```python
from build123d import *

# Parameters (mm, degrees)
F0_W     = 125.222
F0_H     = 98.425
F0_W_2   = 99.822
F0_H_2   = 85.979
F0_R     = 1.27
F0_R_2   = 36.5125
F1_DEPTH = 19.05
F2_W     = 559.8626548463
F2_H     = 85.725
F3_DEPTH = 12.7
F2_W_2   = 125.222
F2_R     = 1.27
F2_R_2   = 36.5125
F4_DEPTH = 12.7


with BuildPart() as f1:
    # F0 (on Front) → F1 (new body)
    with BuildSketch(Plane.XZ):
        with Locations((-326.1520862579, 56.1317810915)):
            Rectangle(F0_W, F0_H)
        with Locations((-326.1520862579, 56.1317810915)):
            Rectangle(F0_W_2, F0_H_2, mode=Mode.SUBTRACT)
        with Locations((-326.1520862579, 56.1317810915)):
            Rectangle(F0_W_2, F0_H_2)
        with Locations((-372.7610862579, 16.7490810915)):
            Circle(F0_R, mode=Mode.SUBTRACT)
        with Locations((-279.5430862579, 16.7617810915)):
            Circle(F0_R, mode=Mode.SUBTRACT)
        with Locations((-326.1520862579, 56.1317810915)):
            Circle(F0_R_2, mode=Mode.SUBTRACT)
        with Locations((-372.7610862579, 95.4890810915)):
            Circle(F0_R, mode=Mode.SUBTRACT)
        with Locations((-279.5430871231, 95.5017810915)):
            Circle(F0_R, mode=Mode.SUBTRACT)
    extrude(amount=F1_DEPTH)

    # F2 (on face) → F3 (cut)
    with BuildSketch(Plane.XZ.offset(19.05)):
        with Locations((-149.6497262269, 56.1317810915)):
            Rectangle(F2_W, F2_H)
    extrude(amount=-F3_DEPTH, mode=Mode.SUBTRACT)

    # F2 (on face) → F4 (cut)
    with BuildSketch(Plane.XZ.offset(19.05)):
        with Locations((-326.1520862579, 56.1317810915)):
            Rectangle(F2_W_2, F2_H)
        with Locations((-372.7610862579, 16.7490810915)):
            Circle(F2_R, mode=Mode.SUBTRACT)
        with Locations((-279.5430862579, 16.7617810915)):
            Circle(F2_R, mode=Mode.SUBTRACT)
        with Locations((-326.1520862579, 56.1317810915)):
            Circle(F2_R_2, mode=Mode.SUBTRACT)
        with Locations((-372.7610862579, 95.4890810915)):
            Circle(F2_R, mode=Mode.SUBTRACT)
        with Locations((-279.5430871231, 95.5017810915)):
            Circle(F2_R, mode=Mode.SUBTRACT)
    extrude(amount=-F4_DEPTH, mode=Mode.SUBTRACT)


solid = f1.part
```
Geometry check sheet. Reference: the model listing, model coordinates, mm. A direction names the side the tool comes from. Give positions to 0.01 mm unless a question says otherwise; leave off trailing zeros. Write each loop counter-clockwise with the first axis right and the second up, starting at its lowest first coordinate (ties: lowest second). Pieces come first, ordered by that corner, then holes. Notation, with made-up numbers: (-29.75, 12.25) - (-25.75, 12.25) arc R27 ccw to (-25.75, 31.25) - close; hole circle Ø9 at (30, 0). An arc over 180 degrees is marked (long way). Use a Markdown table: item, result.
Q1. Section check B-B, the plane z = 78. Enter the section's corners in (x, y), then the cut area to 3 significant figures.
Computed:
| item | result |
|---|---|
| outline | (-388.76, -6.35) - (-355.39, -6.35) - (-355.39, 0) - (-388.76, 0) - close; (-296.91, -6.35) - (-263.54, -6.35) - (-263.54, 0) - (-296.91, 0) - close |
| area | 424 mm² |
Q2. Section check C-C, the plane x = -303.5. Enter the section's corners in (y, z), then the cut area to 3 significant figures.
Computed:
| item | result |
|---|---|
| outline | (-19.05, 6.92) - (0, 6.92) - (0, 27.5) - (-6.35, 27.5) - (-6.35, 13.27) - (-19.05, 13.27) - close; (-19.05, 98.99) - (-6.35, 98.99) - (-6.35, 84.77) - (0, 84.77) - (0, 105.34) - (-19.05, 105.34) - close |
| area | 423 mm² |
Q3. Draft check along X on faces 3 (the face through (-292.424, -3.131, 42.147)), 4 (the face through (-388.763, -5, 55)), 5 (the face through (-327, -19.05, 102)). Enter one of: pulls with the +X half, pulls with the -X half, needs draft (parallel to the pull), parting line crosses it, or undercut.
Computed:
| item | result |
|---|---|
| face 3 | undercut |
| face 4 | pulls with the -X half |
| face 5 | needs draft |
Q4. Thickness scan on L1, parallel to Z at x = -322, y = -9.5; L2, parallel to X at y = -5.5, z = 16; L3, parallel to Y at x = -271.5, z = 95. Record the ranges inside material, lowest first. Write a range as [from, to].
Computed:
| item | result |
|---|---|
| L1 | z = [6.92, 13.27], [98.99, 105.34] |
| L2 | x = [-388.76, -373.79], [-371.74, -280.56], [-278.53, -263.54] |
| L3 | y = [-6.35, 0] |
Q5. Go/stop test with flat-tipped pins: P1, Ø3, axis at y = -9, z = 72.5, coming from the -X side; P2, Ø8, axis at x = -371, z = 21, coming from the -Y side. Record where each tip stops, or that it passes through.
Computed:
| item | result |
|---|---|
| P1 | passes through |
| P2 | stops at y = -6.35 |
Q6. Set-up check for faces 1 (the face through (-327, -13, 13.269)), 2 (the face through (-327, -19.05, 10)): record each of +Z, -Z, +X, -X, +Y, -Y from which the full face is reachable in a straight line by a thin tool's end or side.
Computed:
| item | result |
|---|---|
| face 1 | +X, -X, -Y |
| face 2 | +Z, -Z, +X, -X, -Y |
Q7. Section check A-A, the plane y = -17.5. Enter the section's corners in (x, z).
Computed:
| item | result |
|---|---|
| outline | (-388.76, 6.92) - (-263.54, 6.92) - (-263.54, 13.27) - (-388.76, 13.27) - close; (-388.76, 98.99) - (-263.54, 98.99) - (-263.54, 105.34) - (-388.76, 105.34) - close |
Q8. Section check D-D, the plane y = -5. Enter the section's corners in (x, z) (1 decimal), then the cut area to 3 significant figures.
Computed:
| item | result |
|---|---|
| outline | (-388.8, 6.9) - (-263.5, 6.9) - (-263.5, 105.3) - (-388.8, 105.3) - close; hole circle Ø2.5 at (-372.8, 16.7); hole circle Ø2.5 at (-372.8, 95.5); hole circle Ø73 at (-326.2, 56.1); hole circle Ø2.5 at (-279.5, 16.8); hole circle Ø2.5 at (-279.5, 95.5) |
| area | 8,120 mm² |
